from build123d import *

# Parameters (mm, degrees)
SKETCH_1_R           = 13.8
SKETCH_1_R_2         = 4
EXTRUDE_1_DEPTH      = 6.5
EXTRUDE_2_DEPTH      = 13
EXTRUDE_2_DEPTH_BACK = 23
SKETCH_2_R           = 6.25
SKETCH_2_R_2         = 4
EXTRUDE_3_DEPTH      = 8
CHAMFER_1_SIZE       = 0.2


with BuildPart() as part:
    # Эскиз1 → Бобышка-Вытянуть1 (new body)
    with BuildSketch(Plane.XY):
        with Locations(Location((0, 0, 0), (0, 0, 180))):
            Circle(SKETCH_1_R)
        with Locations(Location((0, 0, 0), (0, 0, 180))):
            Circle(SKETCH_1_R_2, mode=Mode.SUBTRACT)
    extrude(amount=EXTRUDE_1_DEPTH)

    # Эскиз2 → Бобышка-Вытянуть2 (add, two sides: drawn at the far end of the back side and taken through both)
    with BuildSketch(Plane.XY.offset(6.5).offset(-EXTRUDE_2_DEPTH_BACK)):
        Circle(SKETCH_2_R)
        with Locations(Location((0, 0, 0), (0, 0, 180))):
            Circle(SKETCH_2_R_2, mode=Mode.SUBTRACT)
    extrude(amount=EXTRUDE_2_DEPTH + EXTRUDE_2_DEPTH_BACK)

    # Эскиз3 → Бобышка-Вытянуть3 (add)
    with BuildSketch(Plane(origin=(0, 0, -16.5), x_dir=(-1, 0, 0), z_dir=(0, 0, -1))):
        with BuildLine():
            Line((-3.464101615, -2), (3.464101615, -2))
            ThreePointArc((3.464101615, -2), (0, -4), (-3.464101615, -2))
        make_face()
    extrude(amount=-EXTRUDE_3_DEPTH)

    # Фаска1
    chamfer_1_edges = [part.edges().sort_by_distance(p)[0] for p in [
        (4, 0, 19.5),
        (-6.25, 0, 19.5),
        (1.03527618, 3.863703305, -16.5),
        (0, -2, -16.5),
    ]]
    chamfer(chamfer_1_edges, length=CHAMFER_1_SIZE)


solid = part.part
Source: CAD feature listing. Evaluate the final solid. Frame: model axes, mm. A direction names the side the tool comes from. Round coordinates to 2 decimals unless told otherwise and drop trailing zeros. Loops run counter-clockwise (first coordinate to the right, second up) from the corner with the lowest first, then second, coordinate; pieces in that order, holes last. Notation, with made-up numbers: (23.5, 31.25) - (29.5, 31.25) arc R26 ccw to (29.5, 61.25) - close; hole circle Ø2 at (42.5, 9). An arc over 180 degrees is marked (long way). Write item = value, one per line. Start each with the question number.
Item 1: Section query B-B on x = 0. Output: boundary loops of the cut face in (y, z), plus the area to 3 significant figures.
Item 2: First-contact query: pin 1 Ø2 at (x, z) = (-1, -14) entering from +Y; pin 2 Ø4 at (x, y) = (6.5, 8) entering from +Z; pin 3 Ø1 at (y, z) = (-4, 5.5) entering from -X. Flat tips, straight axial feed; report the tip coordinate or a pass-through.
Item 3: Section query D-D on z = 2. Output: boundary loops of the cut face in (x, y), plus the area to 3 significant figures.
Item 4: Section query C-C on z = 15. Output: boundary loops of the cut face in (x, y), plus the area to 3 significant figures.
Item 5: Mould query, pull axis X, two halves, no side actions, for faces 1 (the face through (10.17, -9.33, 3.2)), 2 (the face through (0.867, 3.905, 1.251)), 3 (the face through (-6, 3, 6.5)). Classes: released by +X, released by -X, zero draft, split by the parting line, or undercut.
Item 6: Material intervals for line 1 (Y direction, x = 0, z = -1); line 2 (Y direction, x = 0, z = 6); line 3 (Z direction, x = 8.5, y = 3.5), sorted ascending.
Item 7: Reachability of faces 4 (the face through (-6, 3, 0)), 5 (the face through (-1.43, 4.12, 19.5)), 6 (the face through (5.96, 1.88, 12.81)), 7 (the face through (0, -2, -12)), 8 (the face through (0, -3, -16.5)) from +Z, -Z, +X, -X, +Y, -Y: full face, straight path, thin tool, end or side. Return the list, or none.
Item 8: Section query A-A on y = 0. Output: boundary loops of the cut face in (x, z), plus the area to 3 significant figures.
Results list:
q1.outline = (-13.8, 0) - (-6.25, 0) - (-6.25, -16.5) - (-2.2, -16.5) - (-2, -16.3) - (-2, -8.5) - (-4, -8.5) - (-4, 19.3) - (-4.2, 19.5) - (-6.05, 19.5) - (-6.25, 19.3) - (-6.25, 6.5) - (-13.8, 6.5) - close; (4, -16.3) - (4.2, -16.5) - (6.25, -16.5) - (6.25, 0) - (13.8, 0) - (13.8, 6.5) - (6.25, 6.5) - (6.25, 19.3) - (6.05, 19.5) - (4.2, 19.5) - (4, 19.3) - close
q1.area = 276 mm²
q2.pin_1 = 6.25
q2.pin_2 = 6.5
q2.pin_3 = -13.35
q3.outline = circle Ø27.6 at (0, 0); hole circle Ø8 at (0, 0)
q3.area = 548 mm²
q4.outline = circle Ø12.5 at (0, 0); hole circle Ø8 at (0, 0)
q4.area = 72.5 mm²
q5.face_1 = split by the parting line
q5.face_2 = undercut
q5.face_3 = zero draft
q6.line_1 = -6.25 to -4, 4 to 6.25
q6.line_2 = -13.8 to -4, 4 to 13.8
q6.line_3 = 0 to 6.5
q7.face_4 = -Z
q7.face_5 = +Z, +X, -X, +Y, -Y
q7.face_6 = +Z
q7.face_7 = +Z, -Z
q7.face_8 = -Z, +X, -X, +Y, -Y
q8.outline = (-13.8, 0) - (-6.25, 0) - (-6.25, -16.5) - (-4.2, -16.5) - (-4, -16.3) - (-4, 19.3) - (-4.2, 19.5) - (-6.05, 19.5) - (-6.25, 19.3) - (-6.25, 6.5) - (-13.8, 6.5) - close; (4, -16.3) - (4.2, -16.5) - (6.25, -16.5) - (6.25, 0) - (13.8, 0) - (13.8, 6.5) - (6.25, 6.5) - (6.25, 19.3) - (6.05, 19.5) - (4.2, 19.5) - (4, 19.3) - close
q8.area = 260 mm²
